Geometry check sheet. Reference: the model listing, model coordinates, mm. A direction names the side the tool comes from. Round coordinates to 2 decimals unless told otherwise and drop trailing zeros. Write each loop counter-clockwise with the first axis right and the second up, starting at its lowest first coordinate (ties: lowest second). Pieces come first, ordered by that corner, then holes. Notation, with made-up numbers: M -28.75,10 L 12.25,10 A24 ccw 12.25,24 Z; hole C -3.5,29 d1. An arc over 180 degrees is marked long. Answer as CSV lines item,"result". Start each with the question number.
```python
from build123d import *

# Parameters (mm, degrees)
SKETCH_W     = 19.2
SKETCH_H     = 25.21
SKETCH_R     = 0.63
PAD_DEPTH    = 0.635
SKETCH001_W  = 7.7
SKETCH001_H  = 9.3
PAD001_DEPTH = 4.1
FILLET_R     = 0.5
SKETCH002_W  = 8.550769
SKETCH002_H  = 4.773829
POCKET_DEPTH = 2.2


with BuildPart() as part:
    # Sketch → Pad (new body, symmetric)
    with BuildSketch(Plane.XY):
        Rectangle(SKETCH_W, SKETCH_H)
        with Locations((-7.53, 10.53)):
            Circle(SKETCH_R, mode=Mode.SUBTRACT)
        with Locations((7.53, 10.53)):
            Circle(SKETCH_R, mode=Mode.SUBTRACT)
        with Locations((7.53, -10.53)):
            Circle(SKETCH_R, mode=Mode.SUBTRACT)
        with Locations((-7.53, -10.53)):
            Circle(SKETCH_R, mode=Mode.SUBTRACT)
    extrude(amount=PAD_DEPTH, both=True)

    # Sketch001 → Pad001 (new body)
    with BuildSketch(Plane.XY.offset(0.635)):
        with Locations((0, -10.155)):
            Rectangle(SKETCH001_W, SKETCH001_H)
    extrude(amount=PAD001_DEPTH)

    # Fillet
    fillet_edges = [part.edges().sort_by_distance(p)[0] for p in [
        (-3.85, -10.155, 4.735),
        (3.85, -10.155, 4.735),
    ]]
    fillet(fillet_edges, radius=FILLET_R)

    # Sketch002 → Pocket (cut)
    with BuildSketch(Plane.XZ.offset(14.805)):
        with Locations((-0.025621, 2.603407)):
            Rectangle(SKETCH002_W, SKETCH002_H)
        with BuildLine():
            Line((-3.85, 4.735), (-3.85, 3.035))
            ThreePointArc((-3.85, 3.035), (-3.804161, 2.825865), (-3.675049, 2.655075))
            Line((-3.675049, 2.655075), (-3.474951, 2.483878))
            ThreePointArc((-3.3, 2.103953), (-3.345839, 2.313089), (-3.474951, 2.483878))
            Line((-3.3, 2.103953), (-3.3, 1.135))
            ThreePointArc((-3.3, 1.135), (-3.153553, 0.781447), (-2.8, 0.635))
            Line((-2.8, 0.635), (2.8, 0.635))
            ThreePointArc((2.8, 0.635), (3.153553, 0.781447), (3.3, 1.135))
            Line((3.3, 1.135), (3.3, 2.103953))
            ThreePointArc((3.474951, 2.483878), (3.345839, 2.313089), (3.3, 2.103953))
            Line((3.474951, 2.483878), (3.675049, 2.655075))
            ThreePointArc((3.675049, 2.655075), (3.804161, 2.825865), (3.85, 3.035))
            Line((3.85, 3.035), (3.85, 4.735))
            Line((3.85, 4.735), (-3.85, 4.735))
        make_face(mode=Mode.SUBTRACT)
    extrude(amount=-POCKET_DEPTH, mode=Mode.SUBTRACT)


solid = part.part
```
1) Mould release check, pull along Y, two halves, no side actions. Record for faces 1 (the flat face through (0, -12.605, 0)), 2 (the flat face through (0, 0, -0.635)), 3 (the cylindrical face through (-6.93, 10.72, -0.01)): released by +Y, released by -Y, zero draft, split by the parting line, or undercut.
2) Go/stop test with flat-tipped pins: pin 1 (6 mm diameter, centred on x = 5.5, y = 1, fed in from +Z) (3 decimals); pin 2 (3 mm diameter, centred on y = -10, z = 3, fed in from -X); pin 3 (1.1 mm diameter, centred on x = 0.5, y = -14, fed in from -Z) (3 decimals). Record where each tip stops, or that it passes through.
3) Section check D-D, the plane y = -12.25. Record the cut outline in (x, z) (3 decimals), plus the area to 3 significant figures.
4) Section check B-B, the plane y = 10.53. Record the cut outline in (x, z) (3 decimals), plus the area to 3 significant figures.
5) Section check A-A, the plane x = -7.53. Record the cut outline in (y, z) (3 decimals).
6) Access from +Z, -Z, +X, -X, +Y, -Y to the whole of each face (thin tool, end or side, straight path). Record for faces 4 (the flat face through (0, -5.505, 3)), 5 (the flat face through (3.85, -9, 2)), 6 (the flat face through (0, -14, 0.635)), 7 (the flat face through (3.3, -13.7, 1.6)).
7) Section check C-C, the plane z = 0.35. Record the cut outline in (x, y) (3 decimals).
8) Scan lines: line 1 (Y direction, x = -7.53, z = -0.1) (3 decimals); line 2 (Z direction, x = 7.5, y = 8.5) (3 decimals); line 3 (Y direction, x = -0.75, z = 2.2) (3 decimals). Record each from-to range of solid material in increasing order. Write a range as from..to.
Results:
1,face 1,"released by -Y"
1,face 2,"zero draft"
1,face 3,"undercut"
2,pin 1,"stops at z = 0.635"
2,pin 2,"stops at x = -3.85"
2,pin 3,"stops at z = 0.635"
3,outline,"M -9.6,-0.635 L 9.6,-0.635 L 9.6,0.635 L 3.85,0.635 L 3.85,4.235 A0.5 ccw 3.35,4.735 L -3.35,4.735 A0.5 ccw -3.85,4.235 L -3.85,0.635 L -9.6,0.635 Z"
3,area,"55.8 mm^2"
4,outline,"M -9.6,-0.635 L -8.16,-0.635 L -8.16,0.635 L -9.6,0.635 Z; M -6.9,-0.635 L 6.9,-0.635 L 6.9,0.635 L -6.9,0.635 Z; M 8.16,-0.635 L 9.6,-0.635 L 9.6,0.635 L 8.16,0.635 Z"
4,area,"21.2 mm^2"
5,outline,"M -12.605,-0.635 L -11.16,-0.635 L -11.16,0.635 L -12.605,0.635 Z; M -9.9,-0.635 L 9.9,-0.635 L 9.9,0.635 L -9.9,0.635 Z; M 11.16,-0.635 L 12.605,-0.635 L 12.605,0.635 L 11.16,0.635 Z"
6,face 4,"+Z, +X, -X, +Y"
6,face 5,"+Z, +X, +Y, -Y"
6,face 6,"-Z, +X, -X, -Y"
6,face 7,"-Z, +X, -Y"
7,outline,"M -9.6,-12.605 L 9.6,-12.605 L 9.6,12.605 L -9.6,12.605 Z; hole C -7.53,-10.53 d1.26; hole C -7.53,10.53 d1.26; hole C 7.53,-10.53 d1.26; hole C 7.53,10.53 d1.26"
8,line 1,"y = -12.605..-11.16, -9.9..9.9, 11.16..12.605"
8,line 2,"z = -0.635..0.635"
8,line 3,"y = -14.805..-5.505"
